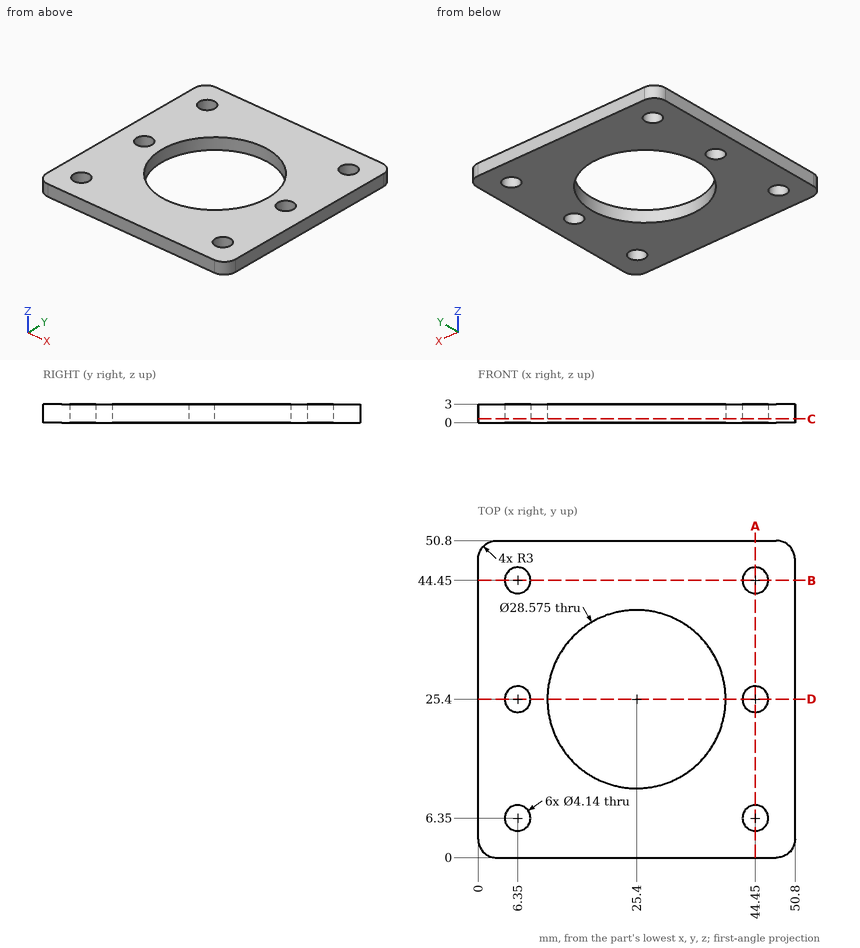
Design review of the part shown in the three views and the two pictorial views. Dimensions are in mm from the part's minimum x, y and z. Round coordinates to 2 decimals unless told otherwise and drop trailing zeros. Order: outer loops, then holes, each group sorted by start corner. A loop starts at its lowest first (then second) coordinate and runs counter-clockwise, first axis right, second up. Notation, with made-up numbers: (44, 68) - (59, 68) arc R18 ccw to (59, 93) - close; hole circle Ø8 at (30.5, -10.75). An arc over 180 degrees is marked (long way). Answer in a Markdown table with one row per item.
(1) Take a section at C-C on z = 0.6. Count the separate pieces of the cut face and the enclosed holes in it, plus the area to 3 significant figures.
Result set:
| item | result |
|---|---|
| separate pieces | 1 |
| enclosed holes | 7 |
| area | 1,850 mm2 |
(2) For line 1 (Y direction, x = 6.35, z = 1.1); line 2 (X direction, y = 6.5, z = 1.4); line 3 (X direction, y = 25.5, z = 1.95), list the stretches that pass through material, from the lowest coordinate up. Write a range as from..to.
Result set:
| item | result |
|---|---|
| line 1 | y = 0..4.28, 8.42..23.33, 27.47..42.38, 46.52..50.8 |
| line 2 | x = 0..4.29, 8.41..42.39, 46.51..50.8 |
| line 3 | x = 0..4.28, 8.42..11.11, 39.69..42.38, 46.52..50.8 |
(3) Take a section at A-A on x = 44.45. Write out the cut boundary in (y, z).
Result set:
| item | result |
|---|---|
| outline | (0, 0) - (4.28, 0) - (4.28, 3) - (0, 3) - close; (8.42, 0) - (23.33, 0) - (23.33, 3) - (8.42, 3) - close; (27.47, 0) - (42.38, 0) - (42.38, 3) - (27.47, 3) - close; (46.52, 0) - (50.8, 0) - (50.8, 3) - (46.52, 3) - close |
(4) Take a section at B-B on y = 44.45. Write out the cut boundary in (x, z).
Result set:
| item | result |
|---|---|
| outline | (0, 0) - (4.28, 0) - (4.28, 3) - (0, 3) - close; (8.42, 0) - (42.38, 0) - (42.38, 3) - (8.42, 3) - close; (46.52, 0) - (50.8, 0) - (50.8, 3) - (46.52, 3) - close |
(5) Take a section at D-D on y = 25.4. Write out the cut boundary in (x, z).
Result set:
| item | result |
|---|---|
| outline | (0, 0) - (4.28, 0) - (4.28, 3) - (0, 3) - close; (8.42, 0) - (11.11, 0) - (11.11, 3) - (8.42, 3) - close; (39.69, 0) - (42.38, 0) - (42.38, 3) - (39.69, 3) - close; (46.52, 0) - (50.8, 0) - (50.8, 3) - (46.52, 3) - close |
